Source: three-view drawing plus pictorial views. Frame: mm from the lowest corner of the part. A direction names the side the tool comes from. Give positions to 0.01 mm unless a question says otherwise; leave off trailing zeros. Order: outer loops, then holes, each group sorted by start corner. A loop starts at its lowest first (then second) coordinate and runs counter-clockwise, first axis right, second up. Notation, with made-up numbers: (-22, 73) -> (37, 73) arc R20 ccw to (37, 84) -> close; hole circle Ø6 at (84, -16). An arc over 180 degrees is marked (long way). Answer in a Markdown table with one row per item.
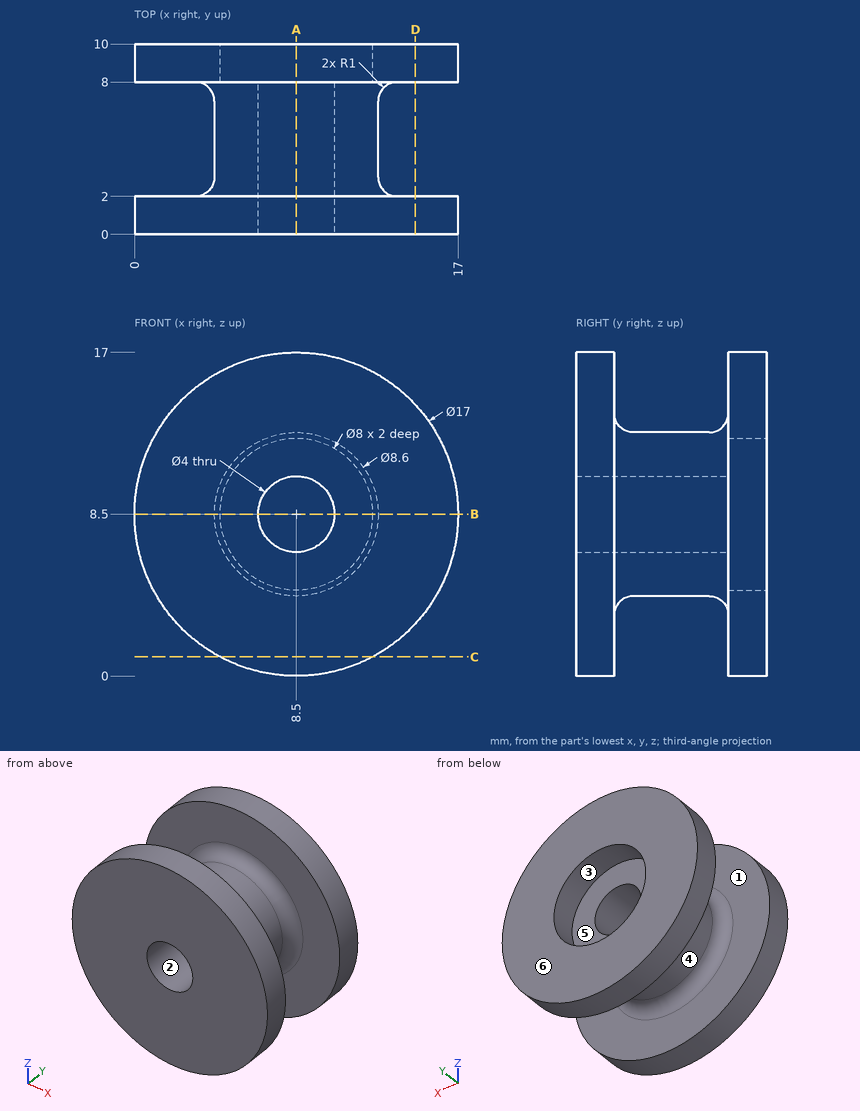
(1) Section query A-A (x = 8.5). Return the cut outline in (y, z).
A:
| item | result |
|---|---|
| outline | (0, 0) -> (2, 0) -> (2, 3.2) arc R1 cw to (3, 4.2) -> (7, 4.2) arc R1 cw to (8, 3.2) -> (8, 0) -> (10, 0) -> (10, 4.5) -> (8, 4.5) -> (8, 6.5) -> (0, 6.5) -> close; (0, 10.5) -> (8, 10.5) -> (8, 12.5) -> (10, 12.5) -> (10, 17) -> (8, 17) -> (8, 13.8) arc R1 cw to (7, 12.8) -> (3, 12.8) arc R1 cw to (2, 13.8) -> (2, 17) -> (0, 17) -> close |
(2) Pull-direction query (X, two-part tool) for the marked faces 4, 5 and 6; classes: +X half, -X half, draft (parallel to the pull), parting line (faces both ways), or undercut.
A:
| item | result |
|---|---|
| face 4 | parting line |
| face 5 | undercut |
| face 6 | draft |
(3) Access query for the marked faces 1, 2 and 3. Directions: +Z, -Z, +X, -X, +Y, -Y. A direction counts if a zero-diameter tool reaches every point of the face in a straight line with its end or side. Return the directions, or none.
A:
| item | result |
|---|---|
| face 1 | none |
| face 2 | +Y, -Y |
| face 3 | +Y |
(4) First-contact query: pin 1 Ø5 at (x, z) = (8.5, 8.5) entering from +Y; pin 2 Ø3 at (y, z) = (8.5, 12) entering from +X. Flat tips, straight axial feed; report the tip coordinate or a pass-through.
A:
| item | result |
|---|---|
| pin 1 | stops at y = 8 |
| pin 2 | stops at x = 16.76 |
(5) Section query B-B (z = 8.5). Return the cut outline in (x, y), plus the area to 3 significant figures.
A:
| item | result |
|---|---|
| outline | (0, 0) -> (6.5, 0) -> (6.5, 8) -> (4.5, 8) -> (4.5, 10) -> (0, 10) -> (0, 8) -> (3.2, 8) arc R1 cw to (4.2, 7) -> (4.2, 3) arc R1 cw to (3.2, 2) -> (0, 2) -> close; (10.5, 0) -> (17, 0) -> (17, 2) -> (13.8, 2) arc R1 cw to (12.8, 3) -> (12.8, 7) arc R1 cw to (13.8, 8) -> (17, 8) -> (17, 10) -> (12.5, 10) -> (12.5, 8) -> (10.5, 8) -> close |
| area | 72.5 mm^2 |
(6) Section query D-D (x = 14.75). Return the cut outline in (y, z), plus the area to 3 significant figures.
A:
| item | result |
|---|---|
| outline | (0, 2.74) -> (2, 2.74) -> (2, 14.26) -> (0, 14.26) -> close; (8, 2.74) -> (10, 2.74) -> (10, 14.26) -> (8, 14.26) -> close |
| area | 46.1 mm^2 |
(7) Section query C-C (z = 1). Return the cut outline in (x, y).
A:
| item | result |
|---|---|
| outline | (4.5, 0) -> (12.5, 0) -> (12.5, 2) -> (4.5, 2) -> close; (4.5, 8) -> (12.5, 8) -> (12.5, 10) -> (4.5, 10) -> close |
(8) Ray query, probe 1 along Y at (x, z) = (12.5, 1.5); probe 2 along Z at (x, y) = (8.5, 6.25). Return the intervals inside material, ascending.
A:
| item | result |
|---|---|
| probe 1 | y = 0 to 2, 8 to 10 |
| probe 2 | z = 4.2 to 6.5, 10.5 to 12.8 |
